```python
from build123d import *

# Parameters (mm, degrees)
F0_W         = 35
F0_H         = 5
F1_DEPTH     = 77.5
F2_T         = -2
F4_DEPTH     = 3
F6_DEPTH     = 2
F7_T1_DEPTH  = 10.0971618345
F8_W         = 111
F8_H         = 5
F9_DEPTH     = 1
F10_W        = 111
F10_H        = 2
F10_H_2      = 3
F11_DEPTH    = 1
F12_T1_DEPTH = 9.5
F13_R        = 0.99999
F14_R        = 0.5
F15_R        = 4
F16_DEPTH    = 1
F17_W        = 2
F17_H        = 10
F18_DEPTH    = 1
F19_R        = 0.99999
F20_R        = 3


# Not quite as in the source:
# - a fillet or chamfer that OpenCascade refuses, or shapes differently, is made with other operations: its cross-section is extruded or revolved along the edge and cut away or added
# - a fillet or chamfer is up to 0.001 mm smaller than in the source, because OpenCascade refuses the exact size


with BuildPart() as f1:
    # F0 (on Right) → F1 (new body, symmetric)
    with BuildSketch(Plane.YZ):
        Rectangle(F0_W, F0_H)
    extrude(amount=F1_DEPTH, both=True)

    # F2
    f2_openings = [f1.faces().sort_by_distance(p)[0] for p in [
        (0, 0, 2.5),
    ]]
    offset(amount=F2_T, openings=f2_openings)

    # F3 (on Front) → F4 (join, symmetric)
    with BuildSketch(Plane.XZ):
        Polygon((-71.5, 2.5), (-75.5, 2.5), (-75.5, 0.5), (-73.5, 0.5), align=None)
    extrude(amount=F4_DEPTH, both=True)

    # F5 (on Front) → F6 (join, symmetric)
    with BuildSketch(Plane.XZ):
        Polygon((81.4, 1), (77.5, 1), (77.5, 0), (79.4, 0), (81.4, 0), align=None)
        Polygon((79.4, -1), (81.4, 0), (79.4, 0), align=None)
    extrude(amount=F6_DEPTH, both=True)

    # F7: fillet of radius 2 on 1 edges, made by hand

    # F7_s2 → F7_t1 (cut)
    with BuildSketch(Plane.XZ.offset(-5.0485809173)):
        with BuildLine():
            ThreePointArc((81.4, 1), (81.0488845703, 0.09023972), (80.3093065335, -0.5453467333))
            Line((80.3093065335, -0.5453467333), (81.4, 0))
            Line((81.4, 0), (81.4, 1))
        make_face()
    extrude(amount=F7_T1_DEPTH, mode=Mode.SUBTRACT)

    # F8 (on face) → F9 (join)
    with BuildSketch(Plane(origin=(0, -15.5, 0), x_dir=(-1, 0, 0), z_dir=(0, 1, 0))):
        with Locations((0, 2)):
            Rectangle(F8_W, F8_H)
    extrude(amount=F9_DEPTH)

    # F10 (on face) → F11 (join)
    with BuildSketch(Plane.XZ.offset(-15.5)):
        with Locations((0, 3.5)):
            Rectangle(F10_W, F10_H)
        with Locations((0, 1)):
            Rectangle(F10_W, F10_H_2)
    extrude(amount=F11_DEPTH)

    # F12: fillet of radius 5 on 2 edges, made by hand

    # F12_s2 → F12_t1 (cut)
    with BuildSketch(Plane.XY.offset(2.5)):
        with BuildLine():
            ThreePointArc((52.5, 15.5), (54.0811388301, 15.2434164903), (55.5, 14.5))
            Line((55.5, 14.5), (55.5, 15.5))
            Line((55.5, 15.5), (52.5, 15.5))
        make_face()
        with BuildLine():
            ThreePointArc((52.5, -15.5), (54.0811388301, -15.2434164903), (55.5, -14.5))
            Line((55.5, -14.5), (55.5, -15.5))
            Line((55.5, -15.5), (52.5, -15.5))
        make_face()
    extrude(amount=F12_T1_DEPTH, mode=Mode.SUBTRACT)

    # F13 (radius 1 in the source; OpenCascade refuses exactly that, so slightly less here)
    f13_edges = [f1.edges().sort_by_distance(p)[0] for p in [
        (-1.5, -15.5, 4.5),
        (-1.5, 15.5, 4.5),
    ]]
    fillet(f13_edges, radius=F13_R)

    # F14
    f14_edges = [f1.edges().sort_by_distance(p)[0] for p in [
        (-71.5, 0, 2.5),
        (-73.5, -3, 2.5),
        (-73.5, 3, 2.5),
    ]]
    fillet(f14_edges, radius=F14_R)

    # F15 (on face) → F16 (cut)
    with BuildSketch(Plane(origin=(0, 0, -2.5), x_dir=(1, 0, 0), z_dir=(0, 0, -1))):
        with Locations((-64.5, 11.5)):
            Circle(F15_R)
        with Locations((-64.5, -11.5)):
            Circle(F15_R)
        with Locations((69.5, -11.5)):
            Circle(F15_R)
        with Locations((69.5, 11.5)):
            Circle(F15_R)
    extrude(amount=-F16_DEPTH, mode=Mode.SUBTRACT)

    # F17 (on face) → F18 (join)
    with BuildSketch(Plane(origin=(0, 0, -2.5), x_dir=(1, 0, 0), z_dir=(0, 0, -1))):
        with Locations((71.5, 0)):
            Rectangle(F17_W, F17_H)
    extrude(amount=F18_DEPTH)

    # F19 (radius 1 in the source; OpenCascade refuses exactly that, so slightly less here)
    f19_edges = [f1.edges().sort_by_distance(p)[0] for p in [
        (71.5, -5, -3.5),
        (72.5, 0, -3.5),
        (71.5, 5, -3.5),
        (70.5, 0, -3.5),
    ]]
    fillet(f19_edges, radius=F19_R)

    # F20
    f20_edges = [f1.edges().sort_by_distance(p)[0] for p in [
        (-77.5, 0, -2.5),
    ]]
    fillet(f20_edges, radius=F20_R)


solid = f1.part
```
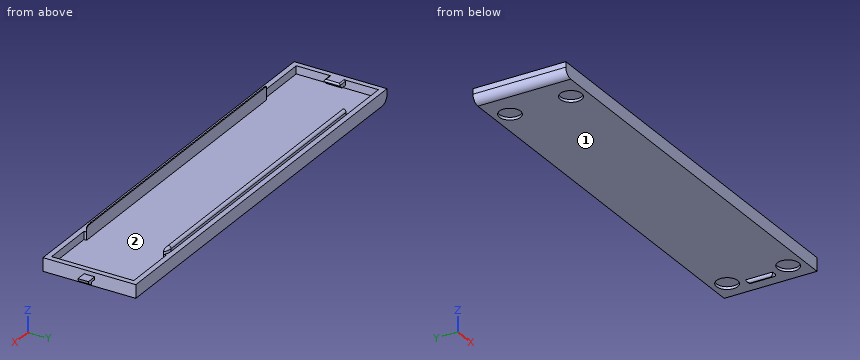
Build history of the part. All positions in model axes, mm. Face numbers are marked on the shaded views. Coordinates: 2 decimals unless noted, no trailing zeros. Order: outer loops, then holes, each group sorted by start corner. A loop starts at its lowest first (then second) coordinate and runs counter-clockwise, first axis right, second up. Notation, with made-up numbers: M 60,-21.75 L 112,-21.75 A20 cw 112,-7.75 Z; hole C 26,57 d3. An arc over 180 degrees is marked long. One line per question, with ' | ' between items. Start each with the question number.
1. Wall check: line 1 along Y through (x, z) = (69.5, -1.7); line 2 along Y through (x, z) = (36, 1.5); line 3 along Y through (x, z) = (-58, 1.25). Give the ranges that are in metal, low to high. Write a range as [from, to].
2. Cut at A-A (x = -64.5). Write the cut outline in (y, z).
3. Flat gauge pins, fed straight in: P1, Ø5, axis at x = 69.5, y = 11.5, coming from the -Z side; P2, Ø3, axis at y = -13, z = 3, coming from the +X side; P3, Ø1, axis at x = 79, z = 0, coming from the +Y side. Where does each tip first touch, or does it go through?
4. Cut at B-B (y = -11.5). Write the cut outline in (x, z), plus the area to 3 significant figures.
5. Mould opens along X. For the marked faces 1 and 2 say: +X half, -X half, draft (parallel to the pull), parting line (faces both ways), or undercut.
The answers:
1) line 1: y = [-17.5, -15.5], [-7.5, 7.5], [15.5, 17.5] | line 2: y = [-17.5, -14.5], [14.5, 17.5] | line 3: y = [-17.5, -15.5], [15.5, 17.5]
2) outline: M -17.5,-2.5 L -15.5,-2.5 L -15.5,-1.5 L -7.5,-1.5 L -7.5,-2.5 L 7.5,-2.5 L 7.5,-1.5 L 15.5,-1.5 L 15.5,-2.5 L 17.5,-2.5 L 17.5,2.5 L 15.5,2.5 L 15.5,-0.5 L -15.5,-0.5 L -15.5,2.5 L -17.5,2.5 Z
3) P1: stops at z = -1.5 | P2: stops at x = 77.5 | P3: stops at y = 2
4) outline: M -77.5,0.5 A3 ccw -74.5,-2.5 L -68.5,-2.5 L -68.5,-1.5 L -60.5,-1.5 L -60.5,-2.5 L 65.5,-2.5 L 65.5,-1.5 L 73.5,-1.5 L 73.5,-2.5 L 77.5,-2.5 L 77.5,2.5 L 75.5,2.5 L 75.5,-0.5 L -75.5,-0.5 L -75.5,2.5 L -77.5,2.5 Z | area: 304 mm2
5) face 1: draft | face 2: undercut
